Verification items for the finished model (mm, model axes). Round coordinates to 2 decimals unless told otherwise and drop trailing zeros. Loops run counter-clockwise (first coordinate to the right, second up) from the corner with the lowest first, then second, coordinate; pieces in that order, holes last. Notation, with made-up numbers: M -35,-39.5 L 13,-39.5 A17 ccw 13,-28.5 Z; hole C 77,11.5 d3. An arc over 180 degrees is marked long. One line per item, written item: value.
Autodesk Inventor part; units mm, degrees
ref_plane "YZ Plane" through (0, 0, 0) normal (1, 0, 0) x (0, 1, 0)
ref_plane "XZ Plane" through (0, 0, 0) normal (0, 1, 0) x (-1, 0, 0)
ref_plane "XY Plane" through (0, 0, 0) normal (0, 0, 1) x (1, 0, 0)
sketch "Sketch1" plane through (0, 0, 0) normal (0, 0, 1) x (1, 0, 0)
  circle A0 centre (0, 0) radius 33
  circle A1 centre (0, 0) radius 17.5
  circle A2 centre (-22.5, 0) radius 2
  circle A3 centre (-15.9099, -15.9099) radius 2
  circle A4 centre (0, -22.5) radius 2
  circle A5 centre (15.9099, -15.9099) radius 2
  circle A6 centre (22.5, 0) radius 2
  circle A7 centre (15.9099, 15.9099) radius 2
  circle A8 centre (0, 22.5) radius 2
  circle A9 centre (-15.9099, 15.9099) radius 2
  dimension "d0" = 66
  dimension "d1" = 35
  dimension "d2" = 4
  dimension "d3" = 22.5
  dimension "d6" = 360
extrude "Extrusion1" add sketch "Sketch1" along normal blind 15
properties part number "Slewing B" material "Aluminum 6061"
(1) Sectioned sample at A-A on y = 0. Enter the section's corners in (x, z), and give its area (3 significant figures).
Completed:
outline: M -33,0 L -24.5,0 L -24.5,15 L -33,15 Z; M -20.5,0 L -17.5,0 L -17.5,15 L -20.5,15 Z; M 17.5,0 L 20.5,0 L 20.5,15 L 17.5,15 Z; M 24.5,0 L 33,0 L 33,15 L 24.5,15 Z
area: 345 mm^2
(2) Sectioned sample at C-C on x = 22.5. Enter the section's corners in (y, z).
Completed:
outline: M -24.14,0 L -2,0 L -2,15 L -24.14,15 Z; M 2,0 L 24.14,0 L 24.14,15 L 2,15 Z
(3) Sectioned sample at D-D on z = 11. Count the separate pieces of the cut face and the enclosed holes in it, and give its area (3 significant figures).
Completed:
separate pieces: 1
enclosed holes: 9
area: 2,360 mm^2
(4) Depth check by flat-ended pin: pin 1 Ø1 at (x, z) = (23, 7.5) entering from +Y; pin 2 Ø4 at (y, z) = (13, 6.5) entering from -X; pin 3 Ø5 at (y, z) = (-6.5, 7.5) entering from -X. Enter the tip coordinate at first touch or a pass-through.
Completed:
pin 1: stops at y = 24.14
pin 2: stops at x = -31.11
pin 3: stops at x = -32.76
(5) Thickness scan on L1, parallel to Y at x = 0, z = 8; L2, parallel to Y at x = 15.5, z = 12.25; L3, parallel to X at y = 1, z = 9.75. Record the ranges inside material, lowest first. Write a range as from..to.
Completed:
L1: y = -33..-24.5, -20.5..-17.5, 17.5..20.5, 24.5..33
L2: y = -29.13..-17.87, -13.95..-8.12, 8.12..13.95, 17.87..29.13
L3: x = -32.98..-24.23, -20.77..-17.47, 17.47..20.77, 24.23..32.98
(6) Mould release check, pull along Y, two halves, no side actions. Record for faces 1 (the face through (-24.1, 1.2, 7.4)), 2 (the face through (30.5, 12.6, 7.4)), 3 (the face through (-14.062, 16.676, 7.395)), 4 (the face through (14, -14, 15)): +Y half, -Y half, draft (parallel to the pull), parting line (faces both ways), or undercut.
Completed:
face 1: undercut
face 2: parting line
face 3: undercut
face 4: draft
